The figure shows three views and two pictorial views of one solid part (mm, origin at its lowest corner). Answer the questions. Give positions to 0.01 mm unless a question says otherwise; leave off trailing zeros. Loops run counter-clockwise (first coordinate to the right, second up) from the corner with the lowest first, then second, coordinate; pieces in that order, holes last. Notation, with made-up numbers: M 88.5,2.5 L 117.5,2.5 A20 cw 117.5,16.5 Z; hole C 26,-28.75 d6. An arc over 180 degrees is marked long. Answer in a Markdown table with one row per item. Add a question column.
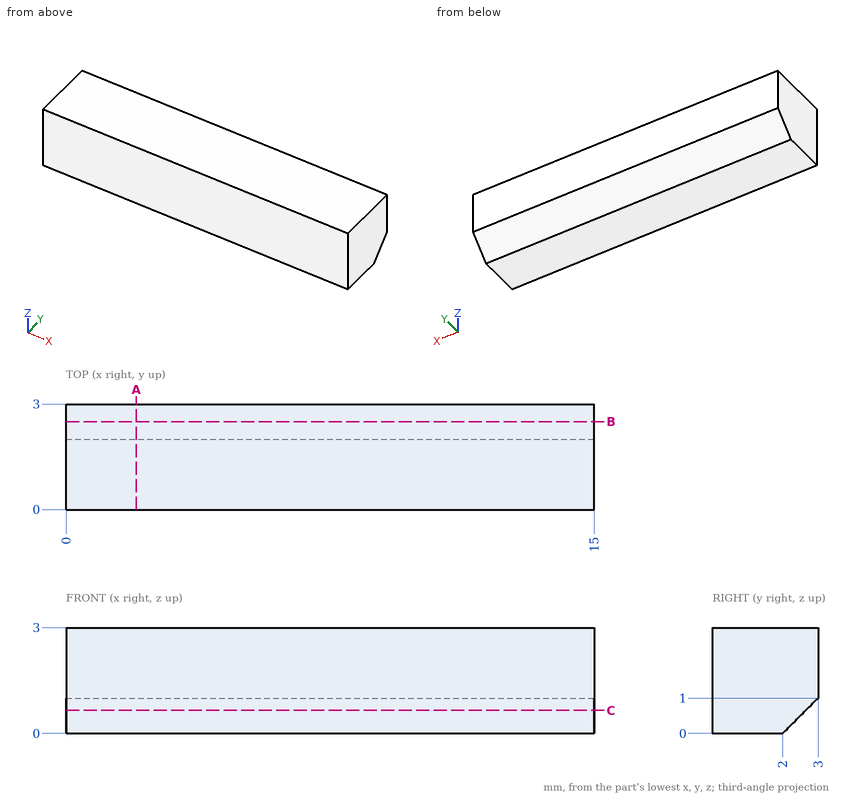
(1) Section A-A, the plane x = 2 is taken. Determine the outline of the cut face in (y, z), and give its area (3 significant figures).
(2) Section C-C, the plane z = 0.65 is taken. Determine the outline of the cut face in (x, y), and give its area (4 significant figures).
(3) Section B-B, the plane y = 2.5 is taken. Determine the outline of the cut face in (x, z), and give its area (3 significant figures).
(4) Consider line 1 along Y through (x, z) = (6.5, 0.25); line 2 along Y through (x, z) = (10.25, 0.55); line 3 along Z through (x, y) = (11, 2.05). Determine where each line is inside the solid, lowest interval first. Write a range as from..to.
Numbers:
| question | item | result |
|---|---|---|
| 1 | outline | M 0,0 L 2,0 L 3,1 L 3,3 L 0,3 Z |
| 1 | area | 8.50 mm² |
| 2 | outline | M 0,0 L 15,0 L 15,2.65 L 0,2.65 Z |
| 2 | area | 39.75 mm² |
| 3 | outline | M 0,0.5 L 15,0.5 L 15,3 L 0,3 Z |
| 3 | area | 37.5 mm² |
| 4 | line 1 | y = 0..2.25 |
| 4 | line 2 | y = 0..2.55 |
| 4 | line 3 | z = 0.05..3 |
